Could you check a few things on this model? Use its own coordinates, in mm. Face numbers are marked on the shaded views. A direction names the side the tool comes from. Coordinates: 2 decimals unless noted, no trailing zeros. Write each loop counter-clockwise with the first axis right and the second up, starting at its lowest first coordinate (ties: lowest second). Pieces come first, ordered by that corner, then holes.
Item 1: Thinking about a two-plate mould opening in Y: for the marked faces 1, 2 and 3, which applies, +Y half, -Y half, draft (parallel to the pull), parting line (faces both ways), or undercut?
Item 2: Which directions (+Z, -Z, +X, -X, +Y, -Y) give clear straight access to the entire face, cutting with the end or side of a thin tool? Please do the marked faces 4 and 5.
Item 3: I want a section at D-D on z = -11.75. Please give me the cut outline in (x, y).
Item 4: I want a section at C-C on y = -3.25. Please give me the cut outline in (x, z) (3 decimals), then the cut area to 3 significant figures.
Item 5: If I drill on probe 1 along Y at (x, z) = (-5.5, -6); probe 2 along Z at (x, y) = (0, 3.9) (3 decimals); probe 3 along Z at (x, y) = (4.5, 0.75), over which ranges is the centre line in solid material (lowest first)?
Item 6: I want a section at A-A on z = -2.5. Please give me the cut outline in (x, y), then the cut area to 3 significant figures.
Item 7: I want a section at B-B on x = 0. Please give me the cut outline in (y, z) (3 decimals).
Item 8: For P1, Ø3.5, axis at x = -1.5, z = -10, coming from the +Y side; P2, Ø1.5, axis at x = 2, z = -6.5, coming from the -Y side; P3, Ø3.5, axis at x = 0, z = -7.825, coming from the -Y side; P4, Ø1, axis at x = 1, y = -1.5, coming from the -Z side, each with a flat end and sliding along its axis, tell me the tip position at first contact or that it passes through.
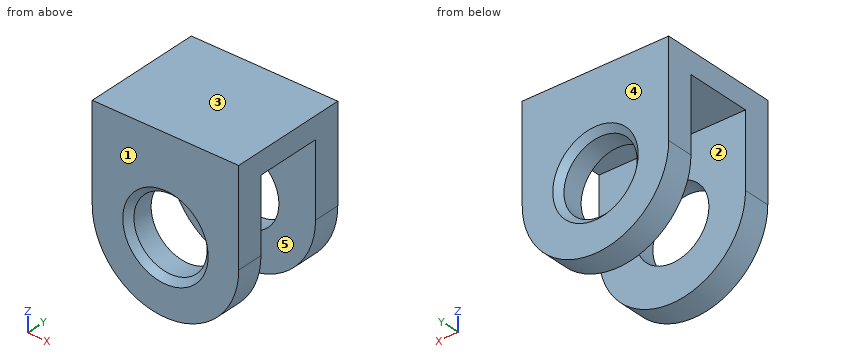
from build123d import *

# Parameters (mm, degrees)
SKETCH1_R           = 3
BOSS_EXTRUDE1_DEPTH = 4.9
CUT_EXTRUDE1_DEPTH  = 2.7
CHAMFER1_SIZE       = 0.5


with BuildPart() as part:
    # Sketch1 → Boss-Extrude1 (new, symmetric)
    with BuildSketch(Plane(origin=(0, 0, 0), x_dir=(1, 0, 0), z_dir=(0, 1, 0))):
        with BuildLine():
            Line((-6, 7.825), (-6, 0))
            Line((-6, 0), (6, 0))
            Line((6, 0), (6, 7.825))
            ThreePointArc((6, 7.825), (0, 13.825), (-6, 7.825))
        make_face()
        with Locations(Location((0, 7.825, 0), (0, 0, 270))):
            Circle(SKETCH1_R, mode=Mode.SUBTRACT)
    extrude(amount=BOSS_EXTRUDE1_DEPTH, both=True)

    # Sketch3 → Cut-Extrude1 (cut, symmetric)
    with BuildSketch(Plane(origin=(0, 0, 0), x_dir=(1, 0, 0), z_dir=(0, 1, 0))):
        with BuildLine():
            Line((6, 1.8), (-6, 1.8))
            Line((-6, 1.8), (-6, 7.825))
            ThreePointArc((-6, 7.825), (0, 13.825), (6, 7.825))
            Line((6, 7.825), (6, 1.8))
        make_face()
    extrude(amount=CUT_EXTRUDE1_DEPTH, both=True, mode=Mode.SUBTRACT)

    # Chamfer1
    chamfer1_edges = [part.edges().sort_by_distance(p)[0] for p in [
        (0, -4.9, -10.825),
        (0, 4.9, -10.825),
    ]]
    chamfer(chamfer1_edges, length=CHAMFER1_SIZE)


solid = part.part
Response values:
1. face 1: -Y half
1. face 2: undercut
1. face 3: draft
2. face 4: +Z, -Z, +X, -X, +Y
2. face 5: -Z, +X, -X
3. outline: (-4.54, -4.9) - (4.54, -4.9) - (4.54, -2.7) - (-4.54, -2.7) - close; (-4.54, 2.7) - (4.54, 2.7) - (4.54, 4.9) - (-4.54, 4.9) - close
4. outline: (-6, -7.825) arc R6 ccw to (6, -7.825) - (6, 0) - (-6, 0) - close; hole circle Ø6 at (0, -7.825)
4. area: 122 mm2
5. probe 1: y = -4.9 to -2.7, 2.7 to 4.9
5. probe 2: z = -13.825 to -10.825, -4.825 to 0
5. probe 3: z = -1.8 to 0
6. outline: (-6, -4.9) - (6, -4.9) - (6, -2.7) - (-6, -2.7) - close; (-6, 2.7) - (6, 2.7) - (6, 4.9) - (-6, 4.9) - close
6. area: 52.8 mm2
7. outline: (-4.9, -13.825) - (-2.7, -13.825) - (-2.7, -10.825) - (-4.4, -10.825) - (-4.9, -11.325) - close; (-4.9, -4.325) - (-4.4, -4.825) - (-2.7, -4.825) - (-2.7, -1.8) - (2.7, -1.8) - (2.7, -4.825) - (4.4, -4.825) - (4.9, -4.325) - (4.9, 0) - (-4.9, 0) - close; (2.7, -13.825) - (4.9, -13.825) - (4.9, -11.325) - (4.4, -10.825) - (2.7, -10.825) - close
8. P1: stops at y = 4.9
8. P2: stops at y = -4.55
8. P3: passes through
8. P4: stops at z = -1.8
